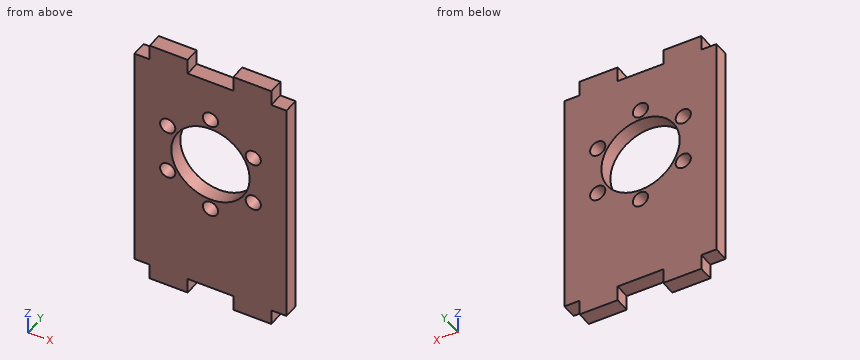
Autodesk Inventor part; units mm, degrees
ref_plane "YZ Plane" through (0, 0, 0) normal (1, 0, 0) x (0, 1, 0)
ref_plane "XZ Plane" through (0, 0, 0) normal (0, 1, 0) x (-1, 0, 0)
ref_plane "XY Plane" through (0, 0, 0) normal (0, 0, 1) x (1, 0, 0)
sketch "Sketch1" plane through (0, 0, 0) normal (0, 1, 0) x (-1, 0, 0)
  circle A0 centre (0, 0) radius 5.15
  line L0 (10, -18) -> (8, -18)
  line L1 (8, -18) -> (8, -20)
  line L2 (8, -20) -> (3, -20)
  line L3 (3, -20) -> (3, -18)
  line L4 (3, -18) -> (-3, -18)
  line L5 (-3, -18) -> (-3, -20)
  line L6 (-3, -20) -> (-8, -20)
  line L7 (-8, -20) -> (-8, -18)
  line L8 (-8, -18) -> (-10, -18)
  line L9 (10, -18) -> (10, 12)
  line L10 (-10, -18) -> (-10, 12)
  line L11 (10, 12) -> (8, 12)
  line L12 (8, 12) -> (8, 14)
  line L13 (8, 14) -> (3, 14)
  line L14 (3, 14) -> (3, 12)
  line L15 (3, 12) -> (-3, 12)
  line L16 (-3, 12) -> (-3, 14)
  line L17 (-3, 14) -> (-8, 14)
  line L18 (-8, 14) -> (-8, 12)
  line L19 (-8, 12) -> (-10, 12)
  line L20 (0, 0) -> (0, 6.5)
  circle A1 centre (0, 6.5) radius 1
  circle A2 centre (-5.6292, 3.25) radius 1
  circle A3 centre (-5.6292, -3.25) radius 1
  circle A4 centre (0, -6.5) radius 1
  circle A5 centre (5.6292, -3.25) radius 1
  circle A6 centre (5.6292, 3.25) radius 1
  dimension "d7" = 360
  dimension "d33" = 2
  dimension "d34" = 2
  dimension "d35" = 5
  dimension "d36" = 6
  dimension "d37" = 5
  dimension "d42" = 30
  dimension "d43" = 2
  dimension "d44" = 2
  dimension "d45" = 5
  dimension "d46" = 6
  dimension "d47" = 5
  dimension "d48" = 6.5
  dimension "d49" = 2
  dimension "d52" = 360
extrude "Extrusion1" add sketch "Sketch1" along normal blind 2
properties part number "Motor Mount"
Input: part model. Units: mm. Frame: model coordinates. Give positions to 0.01 mm unless a question says otherwise; leave off trailing zeros. Order: outer loops, then holes, each group sorted by start corner. A loop starts at its lowest first (then second) coordinate and runs counter-clockwise, first axis right, second up. Notation, with made-up numbers: M -20.5,-22 L 26.5,-22 A25 ccw 26.5,2 Z; hole C 73,89 d7. An arc over 180 degrees is marked long. One line per question, with ' | ' between items. Start each with the question number.
1. Section query D-D (x = -4.25). Return the cut outline in (y, z).
2. First-contact query: pin 1 Ø0.6 at (x, y) = (1, 1.5) entering from -Z; pin 2 Ø0.6 at (x, y) = (-1.5, 1) entering from +Z; pin 3 Ø0.6 at (y, z) = (1.5, -19) entering from +X. Flat tips, straight axial feed; report the tip coordinate or a pass-through.
3. Section query A-A (z = 0). Return the cut outline in (x, y).
4. Section query B-B (y = 1.15). Return the cut outline in (x, z), and give its area (3 significant figures).
5. Section query C-C (x = 5.75). Return the cut outline in (y, z).
6. Material intervals for probe 1 along Z at (x, y) = (0, 1.1); probe 2 along X at (y, z) = (1.4, 6.5); probe 3 along X at (y, z) = (1.8, -4), sorted ascending. Write a range as [from, to].
Here are the results:
1) outline: M 0,-20 L 2,-20 L 2,-2.91 L 0,-2.91 Z; M 0,2.91 L 2,2.91 L 2,14 L 0,14 Z
2) pin 1: z = -18 | pin 2: z = 12 | pin 3: x = 8
3) outline: M -10,0 L -5.15,0 L -5.15,2 L -10,2 Z; M 5.15,0 L 10,0 L 10,2 L 5.15,2 Z
4) outline: M -10,-18 L -8,-18 L -8,-20 L -3,-20 L -3,-18 L 3,-18 L 3,-20 L 8,-20 L 8,-18 L 10,-18 L 10,12 L 8,12 L 8,14 L 3,14 L 3,12 L -3,12 L -3,14 L -8,14 L -8,12 L -10,12 Z; hole C -5.63,-3.25 d2; hole C -5.63,3.25 d2; hole C 0,0 d10.3; hole C 0,-6.5 d2; hole C 0,6.5 d2; hole C 5.63,-3.25 d2; hole C 5.63,3.25 d2 | area: 538 mm²
5) outline: M 0,-20 L 2,-20 L 2,-4.24 L 0,-4.24 Z; M 0,-2.26 L 2,-2.26 L 2,2.26 L 0,2.26 Z; M 0,4.24 L 2,4.24 L 2,14 L 0,14 Z
6) probe 1: [-18, -7.5], [-5.5, -5.15], [5.15, 5.5], [7.5, 12] | probe 2: [-10, -1], [1, 10] | probe 3: [-10, -6.29], [-4.97, -3.24], [3.24, 4.97], [6.29, 10]
